Design review of the part built by this model. Coordinates are the model's own, in mm. A direction names the side the tool comes from. Give positions to 0.01 mm unless a question says otherwise; leave off trailing zeros. Loops run counter-clockwise (first coordinate to the right, second up) from the corner with the lowest first, then second, coordinate; pieces in that order, holes last. Notation, with made-up numbers: M 83.5,-35 L 89.5,-35 A22 cw 89.5,-29 Z; hole C 12.25,83.5 d5. An arc over 180 degrees is marked long. Answer as CSV lines item,"result".
```python
from build123d import *

# Parameters (mm, degrees)
SKETCH1_W           = 4.6
SKETCH1_H           = 6
SKETCH1_R           = 0.85
EXTRUDE1_DEPTH      = 32
EXTRUDE2_DEPTH      = 1.25
SKETCH3_R           = 0.85
EXTRUDE4_DEPTH      = 8
FILLET2_R           = 1
SKETCH_W            = 4
SKETCH_H            = 2
EXTRUDE5_DEPTH      = 4.6
EXTRUDE5_DEPTH_BACK = 4.6
SKETCH4_W           = 2
SKETCH4_H           = 4
EXTRUDE6_DEPTH      = 3.3
EXTRUDE6_DEPTH_BACK = 3.3


with BuildPart() as part:
    # Sketch1 → Extrude1 (new body)
    with BuildSketch(Plane(origin=(0, 0, 0), x_dir=(1, 0, 0), z_dir=(0, 1, 0))):
        Rectangle(SKETCH1_W, SKETCH1_H)
        with Locations(Location((0, 0, 0), (0, 0, 270))):  # turned: the seam where the file's is
            Circle(SKETCH1_R, mode=Mode.SUBTRACT)
    extrude(amount=EXTRUDE1_DEPTH)

    # Sketch2 → Extrude2 (add, symmetric)
    with BuildSketch(Plane(origin=(0, 0, 0), x_dir=(0, 0, -1), z_dir=(1, 0, 0))):
        Polygon((-3, 25), (-3, 31), (-4, 30), (-4, 26), align=None)
        Polygon((3, 31), (3, 25), (4, 26), (4, 30), align=None)
        Polygon((-4, 2), (-3, 1), (-3, 7), (-4, 6), align=None)
        Polygon((4, 6), (3, 7), (3, 1), (4, 2), align=None)
    extrude(amount=EXTRUDE2_DEPTH, both=True)

    # Sketch3 → Extrude4 (cut, through all)
    with BuildSketch(Plane.XY.offset(3)):
        with Locations((0, 20)):
            Circle(SKETCH3_R)
        with Locations((0, 12)):
            Circle(SKETCH3_R)
    extrude(amount=-EXTRUDE4_DEPTH, mode=Mode.SUBTRACT)

    # Fillet2
    fillet2_edges = [part.edges().sort_by_distance(p)[0] for p in [
        (-2.3, 16, -3),
        (2.3, 16, -3),
        (2.3, 16, 3),
        (-2.3, 16, 3),
    ]]
    fillet(fillet2_edges, radius=FILLET2_R)

    # Sketch → Extrude5 (cut, two sides)
    with BuildSketch(Plane(origin=(0, 0, 0), x_dir=(0, 0, -1), z_dir=(1, 0, 0))) as extrude5_sk:
        with Locations((0, 28)):
            Rectangle(SKETCH_W, SKETCH_H)
        with Locations((0, 4)):
            Rectangle(SKETCH_W, SKETCH_H)
    extrude(amount=EXTRUDE5_DEPTH, mode=Mode.SUBTRACT)
    extrude(extrude5_sk.sketch, amount=-EXTRUDE5_DEPTH_BACK, mode=Mode.SUBTRACT)

    # Sketch4 → Extrude6 (cut, two sides)
    with BuildSketch(Plane(origin=(0, 0, 0), x_dir=(0, 0, -1), z_dir=(1, 0, 0))) as extrude6_sk:
        with Locations((0, 20)):
            Rectangle(SKETCH4_W, SKETCH4_H)
        with Locations((0, 12)):
            Rectangle(SKETCH4_W, SKETCH4_H)
    extrude(amount=EXTRUDE6_DEPTH, mode=Mode.SUBTRACT)
    extrude(extrude6_sk.sketch, amount=-EXTRUDE6_DEPTH_BACK, mode=Mode.SUBTRACT)


solid = part.part
```
1. We need section C-C, the plane y = 28. Write out the cut boundary in (x, z), plus the area to 3 significant figures.
Answer block:
outline,"M -2.3,-2 A1 ccw -1.3,-3 L -1.25,-3 L -1.25,-4 L 1.25,-4 L 1.25,-3 L 1.3,-3 A1 ccw 2.3,-2 Z; M -2.3,2 L 2.3,2 A1 ccw 1.3,3 L 1.25,3 L 1.25,4 L -1.25,4 L -1.25,3 L -1.3,3 A1 ccw Z"
area,"13.3 mm²"
2. We need section B-B, the plane z = 1.5. Write out the cut boundary in (x, y), plus the area to 3 significant figures.
Answer block:
outline,"M -2.3,0 L 2.3,0 L 2.3,3 L -2.3,3 Z; M -2.3,5 L 2.3,5 L 2.3,27 L -2.3,27 Z; M -2.3,29 L 2.3,29 L 2.3,32 L -2.3,32 Z; hole C 0,12 d1.7; hole C 0,20 d1.7"
area,"124 mm²"
3. We need section D-D, the plane x = 0. Count the separate pieces of the cut face and the enclosed holes in it, plus the area to 3 significant figures.
Answer block:
separate pieces,"6"
enclosed holes,"0"
area,"132 mm²"
4. The part is to be moulded in two halves that separate along X. For faces 1 (the flat face through (-1.25, 28, -3.5)), 2 (the flat face through (1.25, 28, 3.5)), 3 (the flat face through (0, 28, -4)), 4 (the cylindrical face through (-0.83, 7.46, -0.18)), say which applies: pulls with the +X half, pulls with the -X half, needs draft (parallel to the pull), parting line crosses it, or undercut.
Answer block:
face 1,"pulls with the -X half"
face 2,"pulls with the +X half"
face 3,"needs draft"
face 4,"undercut"
5. We need section A-A, the plane y = 20. Write out the cut boundary in (x, z), plus the area to 3 significant figures.
Answer block:
outline,"M -2.3,-2 A1 ccw -1.3,-3 L -0.85,-3 L -0.85,-1 L -2.3,-1 Z; M -2.3,1 L -0.85,1 L -0.85,3 L -1.3,3 A1 ccw -2.3,2 Z; M 0.85,-3 L 1.3,-3 A1 ccw 2.3,-2 L 2.3,-1 L 0.85,-1 Z; M 0.85,1 L 2.3,1 L 2.3,2 A1 ccw 1.3,3 L 0.85,3 Z"
area,"10.7 mm²"
6. To check wall thickness, follow L1, parallel to Y at x = 1.05, z = -0.75; L2, parallel to Y at x = -1.05, z = -1.5; L3, parallel to Y at x = 0, z = -2.6. State the ranges of each line that lie inside material, in increasing order. Write a range as [from, to].
Answer block:
L1,"[0, 3], [5, 10], [14, 18], [22, 27], [29, 32]"
L2,"[0, 3], [5, 27], [29, 32]"
L3,"[0, 11.15], [12.85, 19.15], [20.85, 32]"
7. For P1, Ø2, axis at x = 0, y = 20, coming from the -Z side; P2, Ø0.8, axis at y = 28, z = 3.5, coming from the +X side, all flat-tipped, find the tip position at first contact; note any pin that passes through.
Answer block:
P1,"z = -3"
P2,"x = 1.25"
8. For faces 5 (the flat face through (0, 6.5, 3.5)), 6 (the flat face through (0, 6.5, -3.5)), 7 (the cylindrical face through (1.999, 16.224, 2.715)), 8 (the flat face through (0, 4, -2)), 9 (the flat face through (-1.25, 4, 3.5)), list the 3-axis set-ups (+Z, -Z, +X, -X, +Y, -Y) from which the entire face can be reached by the end or side of a thin tool; tool diameter is ignored.
Answer block:
face 5,"+Z, +X, -X"
face 6,"-Z, +X, -X"
face 7,"+Z, +X, +Y, -Y"
face 8,"+X, -X"
face 9,"+Z, -X, +Y, -Y"
